from build123d import *

# Parameters (mm, degrees)
F2_R            = 3
F4_D            = 6.8
F4_DEPTH        = 50.001
F5_R            = 5.5
F6_DEPTH        = 15.001
F6_COPIES_COUNT = 3
F7_SIZE         = 0.5


# Not quite as in the source:
# - a pattern or mirror of a feature is missing from the dataset's text; its kind, count and spacing are read off the source's solid


with BuildPart() as f1:
    # F0 (on Front) → F1 (revolve)
    with BuildSketch(Plane.XZ):
        Polygon((-15, 4), (-15, 50), (-25, 50), (-25, 15), (-50, 15), (-50, 0), (-20, 0), (-20, 4), align=None)
    revolve(axis=Axis((0, 0, 33.7237479181), (0, 0, 1)))

    # F2
    f2_edges = [f1.edges().sort_by_distance(p)[0] for p in [
        (25, 0, 15),
    ]]
    fillet(f2_edges, radius=F2_R)

    # F4 (through all, one way)
    with BuildSketch(Plane(origin=(0, 0, 0), x_dir=(0, 1, 0), z_dir=(-1, 0, 0))):
        with Locations((0, -40)):
            Circle(F4_D / 2)
    extrude(amount=-F4_DEPTH, mode=Mode.SUBTRACT)

    # F5 (on face) → F6 (cut, through all)
    with BuildSketch(Plane.XY.offset(15)):
        with Locations((0, 40)):
            Circle(F5_R)
    f6 = extrude(amount=-F6_DEPTH, mode=Mode.SUBTRACT)

    # F6_copies: F6 ×3 about axis
    f6_copies_axis = Axis((0, 0, 0), (0, 0, 1))
    for i in range(1, F6_COPIES_COUNT):
        add(f6.rotate(f6_copies_axis, i * 360 / F6_COPIES_COUNT), mode=Mode.SUBTRACT)

    # F7
    f7_edges = [f1.edges().sort_by_distance(p)[0] for p in [
        (25, 0, 50),
    ]]
    chamfer(f7_edges, length=F7_SIZE)


solid = f1.part
Input: part model. Units: mm. Frame: model coordinates. A direction names the side the tool comes from. Give positions to 0.01 mm unless a question says otherwise; leave off trailing zeros. Write each loop counter-clockwise with the first axis right and the second up, starting at its lowest first coordinate (ties: lowest second). Pieces come first, ordered by that corner, then holes.
Q1. Set-up query: faces 4 (the face through (4.336, 19.524, 2.028)), 5 (the face through (22, 22, 15)), 6 (the face through (39.72, -22.11, 7.6)), 7 (the face through (19.73, -0.44, 36.63)). Return all of +Z, -Z, +X, -X, +Y, -Y with unobstructed straight access to the full face (end or side cutting, diameter ignored); none if empty.
Q2. Pull-direction query (Y, two-part tool) for faces 1 (the face through (-47.69, -15.02, 7.4)), 2 (the face through (-11, 11, 50)), 3 (the face through (-13.856, 5.745, 27.322)); classes: pulls with the +Y half, pulls with the -Y half, needs draft (parallel to the pull), parting line crosses it, or undercut.
Q3. Section A-A, the plane z = 21.5. Output: boundary loops of the cut face in (x, y).
Q4. First-contact query: P1, Ø6, axis at y = 0, z = 40, coming from the +X side; P2, Ø4, axis at y = 23, z = 5, coming from the -X side; P3, Ø5, axis at x = -9.5, y = -34.5, coming from the +Z side. Flat tips, straight axial feed; report the tip coordinate or a pass-through.
Q5. Section C-C, the plane z = 11.5. Output: boundary loops of the cut face in (x, y).
Q6. Section B-B, the plane y = 37. Output: boundary loops of the cut face in (x, z).
Q7. Material intervals for probe 1 along Y at (x, z) = (0, 3.1); probe 2 along Y at (x, z) = (0, 8); probe 3 along Y at (x, z) = (20, 40), sorted ascending.
Q8. Section D-D, the plane y = -43. Output: boundary loops of the cut face in (x, z), plus the area to 3 significant figures.
Filled in:
1. face 4: -Z
1. face 5: +Z
1. face 6: +Z, -Z
1. face 7: +X
2. face 1: parting line crosses it
2. face 2: needs draft
2. face 3: undercut
3. outline: circle Ø50 at (0, 0); hole circle Ø30 at (0, 0)
4. P1: stops at x = -14.7
4. P2: stops at x = -45.38
4. P3: stops at z = 15
5. outline: circle Ø100 at (0, 0); hole circle Ø11 at (-34.64, -20); hole circle Ø30 at (0, 0); hole circle Ø11 at (0, 40); hole circle Ø11 at (34.64, -20)
6. outline: (-33.63, 0) - (-4.61, 0) - (-4.61, 15) - (-33.63, 15) - close; (4.61, 0) - (33.63, 0) - (33.63, 15) - (4.61, 15) - close
7. probe 1: y = -50 to -20, 20 to 34.5, 45.5 to 50
7. probe 2: y = -50 to -15, 15 to 34.5, 45.5 to 50
7. probe 3: y = -15 to -3.4, 3.4 to 15
8. outline: (-25.51, 0) - (25.51, 0) - (25.51, 15) - (-25.51, 15) - close
8. area: 765 mm2
